The model under review builds one solid part; all positions refer to its coordinate system, in mm. Face numbers are marked on the shaded views. A direction names the side the tool comes from. Coordinates: 2 decimals unless noted, no trailing zeros. Order: outer loops, then holes, each group sorted by start corner. A loop starts at its lowest first (then second) coordinate and runs counter-clockwise, first axis right, second up. Notation, with made-up numbers: (65, 78) -> (97, 78) arc R26 cw to (97, 107) -> close; hole circle Ø3 at (-15.5, 51.25). An arc over 180 degrees is marked (long way). Use one line per item in the form item = value.
from build123d import *

# Parameters (mm, degrees)
CHANFREIN1_SIZE         = 0.4
ESQUISSE2_OUTSIDE_W     = 13.828
ESQUISSE2_OUTSIDE_H     = 13.828
ENL_V_MAT_EXTRU_1_DEPTH = 11.002249747
CHANFREIN2_SIZE         = 0.2
CONG_2_R                = 0.1


with BuildPart() as part:
    # Esquisse1 → Révolution1 (revolve)
    with BuildSketch(Plane.XY, mode=Mode.PRIVATE) as r_volution1_sk:
        with BuildLine():
            Line((0, -6.5), (-1.5, -6.5))
            Line((-1.5, -6.5), (-1.5, 0))
            Line((-1.5, 0), (-4.05, 0))
            Line((-4.05, 0), (-4.05, 1.5))
            ThreePointArc((-4.05, 1.5), (-2.931315388, 1.73386291), (-2, 2.396281786))
            Line((-2, 2.396281786), (-2, 3.746281786))
            ThreePointArc((-2, 3.746281786), (-2.832207881, 6.094635769), (-1.5, 8.2))
            Line((-1.5, 8.2), (0, 8.2))
            Line((0, 8.2), (0, -6.5))
        make_face()
    revolve(r_volution1_sk.sketch.rotate(Axis((0, -9.21016139, 0), (0, 1, 0)), 270), axis=Axis((0, -9.21016139, 0), (0, 1, 0)))

    # Chanfrein1
    # the kernel refuses this chamfer: 0.4 mm, written as the material it takes off along each edge
    with BuildSketch(Plane(origin=(0, 1.5, 0), x_dir=(0, 0, -1), z_dir=(1, 0, 0))) as chanfrein1_piece_1:
        with BuildLine():
            Line((4.05, -CHANFREIN1_SIZE), (3.616082015, 0.033917985))
            ThreePointArc((3.616082015, 0.033917985), (3.826287877, 0.008975254), (4.05, 0))
            Line((4.05, 0), (4.05, -CHANFREIN1_SIZE))
        make_face()
    revolve(axis=Axis((0, 1.5, 0), (0, 1, 0)), mode=Mode.SUBTRACT)

    # Esquisse2 outside → Enlèv. mat.-Extru.1 (cut, through all)
    with BuildSketch(Plane.XZ):
        Rectangle(ESQUISSE2_OUTSIDE_W, ESQUISSE2_OUTSIDE_H)
        Polygon((2.020725942, 3.5), (-2.020725942, 3.5), (-4.041451884, 0), (-2.020725942, -3.5), (2.020725942, -3.5), (4.041451884, 0), align=None, mode=Mode.SUBTRACT)
    extrude(amount=-ENL_V_MAT_EXTRU_1_DEPTH, mode=Mode.SUBTRACT)

    # Chanfrein2
    chanfrein2_edges = [part.edges().sort_by_distance(p)[0] for p in [
        (0, -6.5, 1.5),
    ]]
    chamfer(chanfrein2_edges, length=CHANFREIN2_SIZE)

    # Congé2
    cong_2_edges = [part.edges().sort_by_distance(p)[0] for p in [
        (0, 0, 1.5),
    ]]
    fillet(cong_2_edges, radius=CONG_2_R)


solid = part.part
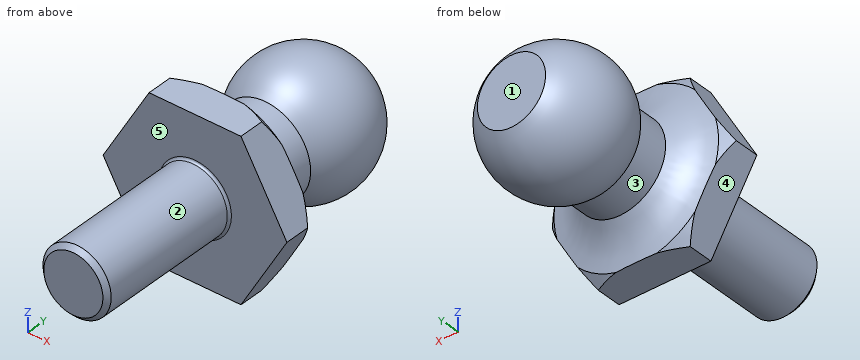
Item 1: Clearance check with flat-ended pins moving along their axes: pin 1 (2 mm diameter, centred on y = 4.5, z = 1.5, fed in from -X); pin 2 (2 mm diameter, centred on y = 1.5, z = -2.5, fed in from -X); pin 3 (4 mm diameter, centred on y = 6, z = 1, fed in from -X). State where each tip first meets the part, or that it passes through.
Results found:
pin_1 = -2.68
pin_2 = -3.18
pin_3 = -2.85
Item 2: To check wall thickness, follow L1, parallel to X at y = -5.25, z = -0.75; L2, parallel to X at y = -3.25, z = 0. State the ranges of each line that lie inside material, in increasing order. Write a range as from..to.
Results found:
L1 = -1.3..1.3
L2 = -1.5..1.5
Item 3: We need section C-C (y = -4.5). Write out the cut boundary in (x, z).
Results found:
outline = circle Ø3 at (0, 0)
Item 4: Draft analysis for pull direction Y (two halves, no side actions). For the marked faces 3, 4 and 5, state which applies: released by +Y, released by -Y, zero draft, split by the parting line, or undercut.
Results found:
face_3 = undercut
face_4 = zero draft
face_5 = released by -Y
Item 5: We need section A-A (x = 0). Write out the cut boundary in (y, z), plus the area to 3 significant figures.
Results found:
outline = (-6.5, -1.3) -> (-6.3, -1.5) -> (-0.1, -1.5) arc R0.1 cw to (0, -1.6) -> (0, -3.5) -> (1.55, -3.5) arc R2.79 cw to (2.4, -2) -> (3.75, -2) arc R2.85 ccw to (8.2, -1.5) -> (8.2, 1.5) arc R2.85 ccw to (3.75, 2) -> (2.4, 2) arc R2.79 cw to (1.55, 3.5) -> (0, 3.5) -> (0, 1.6) arc R0.1 cw to (-0.1, 1.5) -> (-6.3, 1.5) -> (-6.5, 1.3) -> close
area = 62.5 mm²
Item 6: We need section B-B (y = 3). Write out the cut boundary in (x, z).
Results found:
outline = circle Ø4 at (0, 0)
Item 7: Tool access review of the marked faces 1 and 2: name each direction out of +Z, -Z, +X, -X, +Y, -Y from which nothing blocks a thin tool from reaching the whole face with its end or side.
Results found:
face_1 = +Z, -Z, +X, -X, +Y
face_2 = -Y
